Verification items for the finished model (mm, model axes). A direction names the side the tool comes from. Give positions to 0.01 mm unless a question says otherwise; leave off trailing zeros. Order: outer loops, then holes, each group sorted by start corner. A loop starts at its lowest first (then second) coordinate and runs counter-clockwise, first axis right, second up. Notation, with made-up numbers: M -14.75,83.5 L 1.25,83.5 A28 ccw 1.25,112.5 Z; hole C 84,4 d7. An arc over 180 degrees is marked long. Answer as a JSON object with one key per item and string values.
```python
from build123d import *

# Parameters (mm, degrees)
SKETCH1_R                  = 2.2
EXTRUDE_BODY_DEPTH         = 4
SKETCH5_W                  = 10
SKETCH5_H                  = 10
SKETCH5_R                  = 2.2
EXTRUDE_LEGS_DEPTH         = 15
SKETCH6_R                  = 4.215
CUT_BOLT_HEAD_INSETS_DEPTH = 2.5


with BuildPart() as part:
    # Sketch1 → Extrude-Body (new body)
    with BuildSketch(Plane(origin=(0, 0, 0), x_dir=(1, 0, 0), z_dir=(0, 1, 0))):
        with BuildLine():
            Line((10, -10), (10, 10))
            Line((10, 10), (100, 10))
            Line((100, 10), (100, 30))
            Line((100, 30), (90, 30))
            ThreePointArc((90, 30), (50, 21), (10, 30))
            Line((10, 30), (0, 30))
            Line((0, 30), (0, -30))
            Line((0, -30), (10, -30))
            ThreePointArc((10, -30), (50, -21), (90, -30))
            Line((90, -30), (100, -30))
            Line((100, -30), (100, -10))
            Line((100, -10), (10, -10))
        make_face()
        with Locations(Location((5, -12, 0), (0, 0, 270))):
            Circle(SKETCH1_R, mode=Mode.SUBTRACT)
        with Locations(Location((5, 12, 0), (0, 0, 270))):
            Circle(SKETCH1_R, mode=Mode.SUBTRACT)
        with Locations(Location((95, 25, 0), (0, 0, 270))):
            Circle(SKETCH1_R, mode=Mode.SUBTRACT)
        with Locations(Location((95, -25, 0), (0, 0, 270))):
            Circle(SKETCH1_R, mode=Mode.SUBTRACT)
        with Locations(Location((5, 25, 0), (0, 0, 270))):
            Circle(SKETCH1_R, mode=Mode.SUBTRACT)
        with Locations(Location((5, -25, 0), (0, 0, 270))):
            Circle(SKETCH1_R, mode=Mode.SUBTRACT)
    extrude(amount=EXTRUDE_BODY_DEPTH)

    # Sketch5 → Extrude-Legs (add)
    # profile 1 of 4: a face of its own
    with BuildSketch(Plane(origin=(0, 4, 0), x_dir=(1, 0, 0), z_dir=(0, 1, 0))):
        with Locations((95, -25)):
            Rectangle(SKETCH5_W, SKETCH5_H)
        with Locations(Location((95, -25, 0), (0, 0, 270))):
            Circle(SKETCH5_R, mode=Mode.SUBTRACT)
    # profile 2 of 4: a face of its own
    with BuildSketch(Plane(origin=(0, 4, 0), x_dir=(1, 0, 0), z_dir=(0, 1, 0))):
        with Locations((95, 25)):
            Rectangle(SKETCH5_W, SKETCH5_H)
        with Locations(Location((95, 25, 0), (0, 0, 270))):
            Circle(SKETCH5_R, mode=Mode.SUBTRACT)
    # profile 3 of 4: a face of its own
    with BuildSketch(Plane(origin=(0, 4, 0), x_dir=(1, 0, 0), z_dir=(0, 1, 0))):
        with Locations((5, 25)):
            Rectangle(SKETCH5_W, SKETCH5_H)
        with Locations(Location((5, 25, 0), (0, 0, 270))):
            Circle(SKETCH5_R, mode=Mode.SUBTRACT)
    # profile 4 of 4: a face of its own
    with BuildSketch(Plane(origin=(0, 4, 0), x_dir=(1, 0, 0), z_dir=(0, 1, 0))):
        with Locations((5, -25)):
            Rectangle(SKETCH5_W, SKETCH5_H)
        with Locations(Location((5, -25, 0), (0, 0, 270))):
            Circle(SKETCH5_R, mode=Mode.SUBTRACT)
    extrude(amount=EXTRUDE_LEGS_DEPTH)

    # Sketch6 → Cut-Bolt Head Insets (cut)
    with BuildSketch(Plane.XZ):
        with Locations(Location((5, -25, 0), (0, 0, 270))):
            Circle(SKETCH6_R)
        with Locations(Location((5, 25, 0), (0, 0, 270))):
            Circle(SKETCH6_R)
        with Locations(Location((95, 25, 0), (0, 0, 270))):
            Circle(SKETCH6_R)
        with Locations(Location((95, -25, 0), (0, 0, 270))):
            Circle(SKETCH6_R)
    extrude(amount=-CUT_BOLT_HEAD_INSETS_DEPTH, mode=Mode.SUBTRACT)


solid = part.part
```
Q1. Gauge pin test, flat ends, axial feed: pin 1 Ø2.5 at (x, z) = (5, -12) entering from +Y; pin 2 Ø7 at (x, z) = (5, -25) entering from -Y. Record the tip position at first contact, or that the pin passes through.
Resolved:
{"pin 1": "passes through", "pin 2": "stops at y = 2.5"}
Q2. Section check B-B on y = 10.5. Record the cut outline in (x, z), then the cut area to 3 significant figures.
Resolved:
{"outline": "M 0,-30 L 10,-30 L 10,-20 L 0,-20 Z; M 0,20 L 10,20 L 10,30 L 0,30 Z; M 90,-30 L 100,-30 L 100,-20 L 90,-20 Z; M 90,20 L 100,20 L 100,30 L 90,30 Z; hole C 5,-25 d4.4; hole C 5,25 d4.4; hole C 95,-25 d4.4; hole C 95,25 d4.4", "area": "339 mm²"}
Q3. Material ranges on L1, parallel to Z at x = 95, y = 11.75; L2, parallel to X at y = 15, z = 25; L3, parallel to X at y = 3, z = 12, recorded low to high.
Resolved:
{"L1": "z = -30 to -27.2, -22.8 to -20, 20 to 22.8, 27.2 to 30", "L2": "x = 0 to 2.8, 7.2 to 10, 90 to 92.8, 97.2 to 100", "L3": "x = 0 to 2.8, 7.2 to 100"}
Q4. Tool access check on faces 4 (the face through (90, 11, -25)), 5 (the face through (50.6, 2, -21)), 6 (the face through (97.849, 1.232, -21.893)), 7 (the face through (95, 11, 20)). Record the directions out of +Z, -Z, +X, -X, +Y, -Y that give a thin tool (end or side, any length) a straight path to the whole face; none if there is none.
Resolved:
{"face 4": "+Z, -Z, +Y", "face 5": "-Z, +Y, -Y", "face 6": "-Y", "face 7": "+X, -X, +Y"}
Q5. Section check A-A on x = 5. Count the separate pieces of the cut face and the enclosed holes in it, then the cut area to 3 significant figures.
Resolved:
{"separate pieces": "5", "enclosed holes": "0", "area": "317 mm²"}
Q6. Section check D-D on x = 95. Record the cut outline in (y, z) (3 decimals), then the cut area to 3 significant figures.
Resolved:
{"outline": "M 0,-30 L 19,-30 L 19,-27.2 L 2.5,-27.2 L 2.5,-29.215 L 0,-29.215 Z; M 0,-20.785 L 2.5,-20.785 L 2.5,-22.8 L 19,-22.8 L 19,-20 L 4,-20 L 4,-10 L 0,-10 Z; M 0,10 L 4,10 L 4,20 L 19,20 L 19,22.8 L 2.5,22.8 L 2.5,20.785 L 0,20.785 Z; M 0,29.215 L 2.5,29.215 L 2.5,27.2 L 19,27.2 L 19,30 L 0,30 Z", "area": "273 mm²"}
Q7. Section check C-C on z = 12. Record the cut outline in (x, y).
Resolved:
{"outline": "M 0,0 L 2.8,0 L 2.8,4 L 0,4 Z; M 7.2,0 L 100,0 L 100,4 L 7.2,4 Z"}
Q8. Release check for a two-part mould opening along Z. For faces 1 (the face through (10, 2, 0)), 2 (the face through (0, 3, -7)), 3 (the face through (5, 9, -30)) record: +Z half, -Z half, draft (parallel to the pull), parting line (faces both ways), or undercut.
Resolved:
{"face 1": "undercut", "face 2": "draft", "face 3": "-Z half"}
